Work out the finished part from the listing and answer in its coordinate system (mm). A direction names the side the tool comes from. Give positions to 0.01 mm unless a question says otherwise; leave off trailing zeros. Write each loop counter-clockwise with the first axis right and the second up, starting at its lowest first coordinate (ties: lowest second). Pieces come first, ordered by that corner, then holes. Notation, with made-up numbers: (88, -16.5) - (96, -16.5) arc R22 ccw to (96, 12.5) - close; hole circle Ø9 at (86, -38.75). An arc over 180 degrees is marked (long way). Write item = value, one per line.
Autodesk Inventor part; units mm, degrees
ref_plane "YZ Plane" through (0, 0, 0) normal (1, 0, 0) x (0, 1, 0)
ref_plane "XZ Plane" through (0, 0, 0) normal (0, 1, 0) x (-1, 0, 0)
ref_plane "XY Plane" through (0, 0, 0) normal (0, 0, 1) x (1, 0, 0)
sketch "Sketch1" plane through (0, 0, 0) normal (0, 0, 1) x (1, 0, 0)
  line L0 (0, 0) -> (96.52, 0) construction
  line L1 (0, 83.82) -> (0, 96.52)
  line L2 (59.2697, 59.2697) -> (68.2499, 68.2499)
  line L3 (68.2499, 68.2499) -> (59.2697, 59.2697)
  line L4 (0, 83.82) -> (59.2697, 59.2697)
  arc A0 (68.2499, 68.2499) -> (0, 96.52) centre (0, 0) ccw
extrude "Extrusion1" add sketch "Sketch1" along normal mid plane 317.5
sketch "Sketch2" plane through (59.2697, 59.2697, -158.75) normal (-0.3827, -0.9239, 0) x (0.9239, -0.3827, 0)
  circle A0 centre (-32.0765, 57.912) radius 3.175
  line L0 (0, 0) -> (-64.1531, 0)
  circle A1 centre (-32.0765, 217.932) radius 3.175
  point P0 (-32.0765, 158.75)
  dimension "d5" = 6.35
  dimension "d6" = 57.912
  dimension "d7" = 6.35
  dimension "d8" = 160.02
extrude "Extrusion2" cut sketch "Sketch2" against normal blind 7.62
properties part number "Foot2"
1. Find section B-B, the plane x = 45.5. Give the vertices of the cut face in (y, z), then the cut area to 3 significant figures.
Solution:
outline = (64.97, -158.75) - (85.12, -158.75) - (85.12, 158.75) - (64.97, 158.75) - close
area = 6,400 mm^2
2. For a pull along X with two mould halves and no side action, classify faces 1 (the cylindrical face through (30.44, 75.28, -103.94)), 2 (the flat face through (0, 90, -2)), 3 (the flat face through (34, 78, -158.75)) as pulls with the +X half, pulls with the -X half, needs draft (parallel to the pull), parting line crosses it, or undercut.
Solution:
face_1 = undercut
face_2 = pulls with the -X half
face_3 = needs draft
3. Given pin 1 (2 mm diameter, centred on x = 51.5, z = 36, fed in from +Y); pin 2 (2 mm diameter, centred on x = 59, y = 78, fed in from -Z); pin 3 (8 mm diameter, centred on y = 79.5, z = -50, fed in from +X); pin 4 (4 mm diameter, centred on x = 46, z = 81, fed in from -Y), each flat-ended and moving along its own axis, determine where each tip first touches the part or whether it passes through.
Solution:
pin_1 = 82.25
pin_2 = through
pin_3 = 60.13
pin_4 = 63.94
4. A tool of negligible diameter and unlimited length cuts with its end or side. For faces 4 (the flat face through (29.22, 71.717, -2.222)), 5 (the flat face through (32.511, 78.604, -100.794)), from which of +Z, -Z, +X, -X, +Y, -Y can it reach the whole face along a straight path? Write none if from no direction.
Solution:
face_4 = +Z, -Z, -X, -Y
face_5 = none
5. Find section A-A, the plane z = -121. Give the vertices of the cut face in (x, y), then the cut area to 3 significant figures.
Solution:
outline = (0, 83.82) - (59.27, 59.27) - (68.25, 68.25) arc R96.52 ccw to (0, 96.52) - close
area = 1,170 mm^2
6. Straight lines are drawn through the part: line 1 (Y direction, x = 53, z = 95); line 2 (Y direction, x = 40, z = -68.5); line 3 (X direction, y = 79.5, z = 71). For each, find the intervals that lie inside material, in ascending order.
Solution:
line_1 = 61.87 to 80.67
line_2 = 67.25 to 87.84
line_3 = 10.43 to 54.73
